The listing builds one solid part. Answer for the finished solid, in the listing's coordinates (mm). Face numbers are marked on the shaded views. A direction names the side the tool comes from. Round coordinates to 2 decimals unless told otherwise and drop trailing zeros. Write each loop counter-clockwise with the first axis right and the second up, starting at its lowest first coordinate (ties: lowest second). Pieces come first, ordered by that corner, then holes.
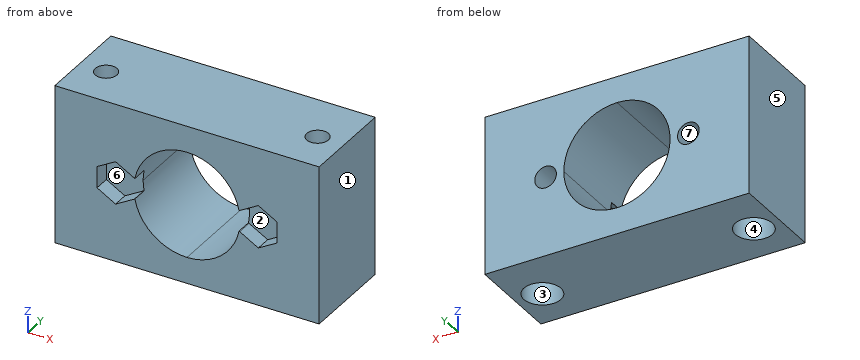
from build123d import *

# Parameters (mm, degrees)
F0_R      = 2.05
F1_DEPTH  = 18
F3_DEPTH  = 30
F4_R      = 3.5
F5_DEPTH  = 5
F7_DEPTH  = 3
F8_R      = 2.05
F9_R      = 2.05
F10_DEPTH = 0.4


with BuildPart() as f1:
    # F0 (on Front) → F1 (new body)
    with BuildSketch(Plane.XZ):
        with BuildLine():
            ThreePointArc((0, 10.05), (7.1064231509, 7.1064231509), (10.05, 0))
            ThreePointArc((10.05, 0), (7.1064231509, -7.1064231509), (0, -10.05))
            Line((0, -10.05), (0, -15))
            Line((0, -15), (25, -15))
            Line((25, -15), (25, 0))
            Line((25, 0), (25, 15))
            Line((25, 15), (0, 15))
            Line((0, 15), (0, 10.05))
        make_face()
        with BuildLine():
            ThreePointArc((15.55, 0), (13.5, -2.05), (11.45, 0))
            ThreePointArc((11.45, 0), (13.5, 2.05), (15.55, 0))
        make_face(mode=Mode.SUBTRACT)
        with BuildLine():
            ThreePointArc((-10.05, 0), (-7.1064231509, 7.1064231509), (0, 10.05))
            Line((0, 10.05), (0, 15))
            Line((0, 15), (-25, 15))
            Line((-25, 15), (-25, 0))
            Line((-25, 0), (-25, -15))
            Line((-25, -15), (0, -15))
            Line((0, -15), (0, -10.05))
            ThreePointArc((0, -10.05), (-7.1064231509, -7.1064231509), (-10.05, 0))
        make_face()
        with Locations((-13.5, 0)):
            Circle(F0_R, mode=Mode.SUBTRACT)
    extrude(amount=F1_DEPTH)

    # F2 (on face) → F3 (cut)
    with BuildSketch(Plane(origin=(0, 0, -15), x_dir=(1, 0, 0), z_dir=(0, 0, -1))):
        with BuildLine():
            ThreePointArc((17.95, 10), (20, 7.95), (22.05, 10))
            Line((22.05, 10), (17.95, 10))
        make_face()
        with BuildLine():
            Line((17.95, 10), (22.05, 10))
            ThreePointArc((22.05, 10), (20, 12.05), (17.95, 10))
        make_face()
        with BuildLine():
            ThreePointArc((-17.95, 10), (-20, 12.05), (-22.05, 10))
            Line((-22.05, 10), (-17.95, 10))
        make_face()
        with BuildLine():
            Line((-17.95, 10), (-22.05, 10))
            ThreePointArc((-22.05, 10), (-20, 7.95), (-17.95, 10))
        make_face()
    extrude(amount=-F3_DEPTH, mode=Mode.SUBTRACT)

    # F4 (on face) → F5 (cut)
    with BuildSketch(Plane(origin=(0, 0, -15), x_dir=(1, 0, 0), z_dir=(0, 0, -1))):
        with Locations((20, 10)):
            Circle(F4_R)
        with Locations((-20, 10)):
            Circle(F4_R)
    extrude(amount=-F5_DEPTH, mode=Mode.SUBTRACT)

    # F6 (on face) → F7 (cut)
    with BuildSketch(Plane.XZ.offset(18)):
        Polygon((-13.5, 4.05), (-13.5, 0), (-13.5, -4.05), (-9.9925971147, -2.025), (-7.9662247081, -0.8550733456), (-7.7903810671, 0.7535499721), (-9.9925971147, 2.025), align=None)
        Polygon((-13.5, -4.05), (-13.5, 0), (-13.5, 4.05), (-17.0074028853, 2.025), (-17.0074028853, -2.025), align=None)
        Polygon((13.5, -4.05), (13.5, 0), (13.5, 4.05), (9.9925971147, 2.025), (9.9925971147, -2.025), align=None)
        Polygon((13.5, 4.05), (13.5, 0), (13.5, -4.05), (17.0074028853, -2.025), (17.0074028853, 2.025), align=None)
        Polygon((9.9925971147, -2.025), (9.9925971147, 2.025), (7.4926645733, 0.5816632743), (7.2557264377, -0.4448669779), align=None)
    extrude(amount=-F7_DEPTH, mode=Mode.SUBTRACT)

    # F8 (on face) + F9 (on face) → F10 (join)
    with BuildSketch(Plane.XZ.offset(15)):
        with Locations((13.5, 0)):
            Circle(F8_R)
    with BuildSketch(Plane.XZ.offset(15)):
        with Locations((-13.5, 0)):
            Circle(F9_R)
    extrude(amount=-F10_DEPTH)


solid = f1.part
1. For a pull along Y with two mould halves and no side action, classify the marked faces 1, 2, 3 and 4 as released by +Y, released by -Y, zero draft, split by the parting line, or undercut.
Geometry says:
face 1: zero draft
face 2: released by -Y
face 3: undercut
face 4: undercut
2. Section A-A on x = -20 is taken. Determine the outline of the cut face in (y, z), plus the area to 4 significant figures.
Geometry says:
outline: (-18, -15) - (-13.5, -15) - (-13.5, -10) - (-12.05, -10) - (-12.05, 15) - (-18, 15) - close; (-7.95, -10) - (-6.5, -10) - (-6.5, -15) - (0, -15) - (0, 15) - (-7.95, 15) - close
area: 402.5 mm2
3. Straight lines are drawn through the part: line 1 along X through (y, z) = (-10, -12.7); line 2 along X through (y, z) = (-16.5, 1.5); line 3 along X through (y, z) = (-11, -3.5). For each, find the intervals that lie inside material, in ascending order.
Geometry says:
line 1: x = -25 to -23.5, -16.5 to 16.5, 23.5 to 25
line 2: x = -25 to -17.01, 17.01 to 25
line 3: x = -25 to -21.79, -18.21 to -9.42, 9.42 to 18.21, 21.79 to 25
4. A tool of negligible diameter and unlimited length cuts with its end or side. For the marked faces 5, 6 and 7, from which of +Z, -Z, +X, -X, +Y, -Y can it reach the whole face along a straight path? Write none if from no direction.
Geometry says:
face 5: +Z, -Z, -X, +Y, -Y
face 6: -Y
face 7: +Y
5. Section C-C on y = -7 is taken. Determine the outline of the cut face in (x, z), plus the area to 3 significant figures.
Geometry says:
outline: (-25, -15) - (-21.8, -15) - (-21.8, -10) - (-18.2, -10) - (-18.2, -15) - (18.2, -15) - (18.2, -10) - (21.8, -10) - (21.8, -15) - (25, -15) - (25, 15) - (-25, 15) - close; hole circle Ø4.1 at (-13.5, 0); hole circle Ø20.1 at (0, 0); hole circle Ø4.1 at (13.5, 0)
area: 1,120 mm2
6. Section B-B on z = -5.25 is taken. Determine the outline of the cut face in (x, y).
Geometry says:
outline: (-25, -18) - (-8.57, -18) - (-8.57, 0) - (-25, 0) - close; (8.57, -18) - (25, -18) - (25, 0) - (8.57, 0) - close; hole circle Ø4.1 at (-20, -10); hole circle Ø4.1 at (20, -10)
7. Given pin 1 (9 mm diameter, centred on x = 20, y = -10, fed in from +Z); pin 2 (3.5 mm diameter, centred on x = -13.5, z = 0, fed in from -Y); pin 3 (1.2 mm diameter, centred on x = -14, z = 0.5, fed in from +Y); pin 4 (3.5 mm diameter, centred on x = -20.5, y = -8.5, fed in from -Z), each flat-ended and moving along its own axis, determine where each tip first touches the part or whether it passes through.
Geometry says:
pin 1: stops at z = 15
pin 2: stops at y = -15
pin 3: stops at y = -14.6
pin 4: stops at z = -10
8. Section D-D on z = 7.75 is taken. Determine the outline of the cut face in (x, y).
Geometry says:
outline: (-25, -18) - (-6.4, -18) - (-6.4, 0) - (-25, 0) - close; (6.4, -18) - (25, -18) - (25, 0) - (6.4, 0) - close; hole circle Ø4.1 at (-20, -10); hole circle Ø4.1 at (20, -10)
